Check sheet for the drawn part. Datum: minimum x, y, z corner. Units: mm. A direction names the side the tool comes from. Round coordinates to 2 decimals unless told otherwise and drop trailing zeros. Write each loop counter-clockwise with the first axis right and the second up, starting at its lowest first coordinate (ties: lowest second). Pieces come first, ordered by that corner, then holes. Notation, with made-up numbers: M 52.5,-29 L 68.5,-29 A28 ccw 68.5,3 Z; hole C 72.25,83 d11. An arc over 180 degrees is marked long. One line per item, written item: value. Start each with the question number.
1. Section check C-C (y = 7.25). Record the boundary of the cut face in (x, z), and give its area (3 significant figures).
2. Section check A-A (z = 98). Record the boundary of the cut face in (x, y).
3. Depth check by flat-ended pin: P1, Ø4, axis at x = 25, y = 18.5, coming from the -Z side; P2, Ø5, axis at x = 66, z = 3.5, coming from the +Y side; P3, Ø0.6, axis at x = 64, y = 2.5, coming from the -Z side; P4, Ø8, axis at x = 28.5, z = 120, coming from the +Y side. Enter the tip coordinate at first touch or a pass-through.
4. Access from +Z, -Z, +X, -X, +Y, -Y to the whole of each face (thin tool, end or side, straight path). Record for the marked faces 1, 2 and 3.
5. Section check D-D (x = 22). Record the boundary of the cut face in (y, z), and give its area (3 significant figures).
6. Scan lines: probe 1 along Y at (x, z) = (22, 114); probe 2 along X at (y, z) = (15.25, 103); probe 3 along Z at (x, y) = (71.5, 19). Record each from-to range of solid material in increasing order. Write a range as [from, to].
7. Section check B-B (x = 70). Record the boundary of the cut face in (y, z).
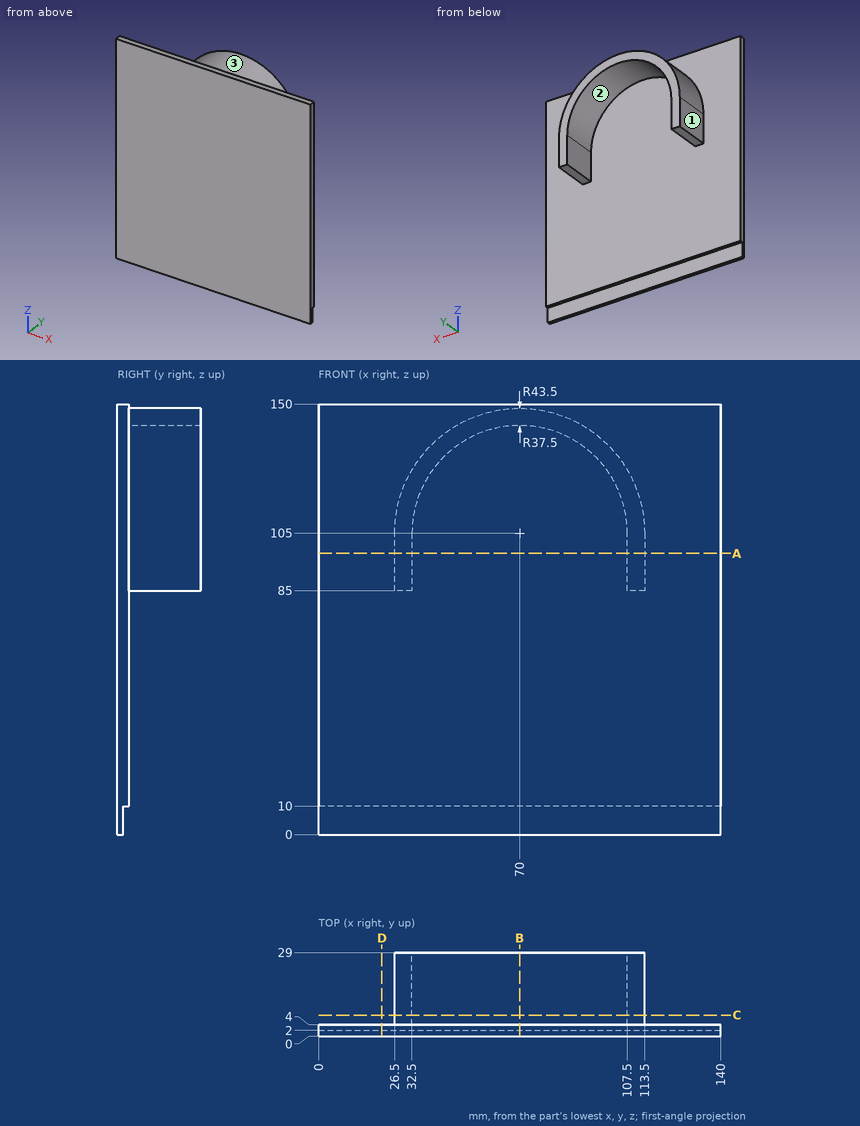
Result sheet:
1. outline: M 26.5,85 L 32.5,85 L 32.5,105 A37.5 cw 107.5,105 L 107.5,85 L 113.5,85 L 113.5,105 A43.5 ccw 26.5,105 Z
1. area: 1,000 mm2
2. outline: M 0,0 L 140,0 L 140,4 L 113.5,4 L 113.5,29 L 107.5,29 L 107.5,4 L 32.5,4 L 32.5,29 L 26.5,29 L 26.5,4 L 0,4 Z
3. P1: stops at z = 85
3. P2: stops at y = 2
3. P3: stops at z = 10
3. P4: stops at y = 29
4. face 1: +Z, -Z, -X, +Y
4. face 2: -Z, +Y
4. face 3: +Z, +Y
5. outline: M 0,0 L 2,0 L 2,10 L 4,10 L 4,150 L 0,150 Z
5. area: 580 mm2
6. probe 1: y = [0, 4]
6. probe 2: x = [26.5, 32.5], [107.5, 113.5]
6. probe 3: z = [142.47, 148.47]
7. outline: M 0,0 L 2,0 L 2,10 L 4,10 L 4,142.5 L 29,142.5 L 29,148.5 L 4,148.5 L 4,150 L 0,150 Z
